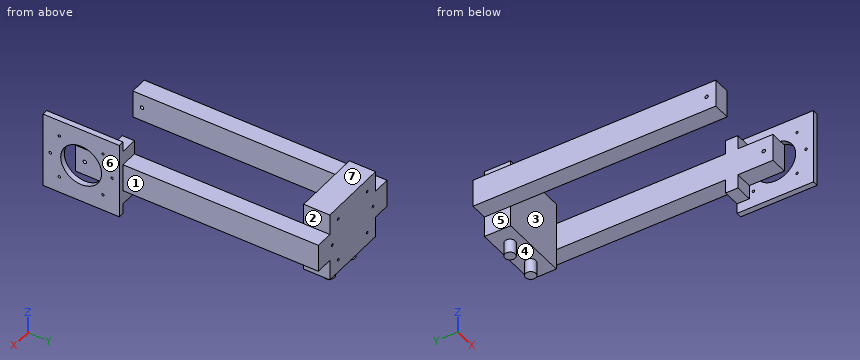
```python
from build123d import *

# Parameters (mm, degrees)
SKETCH_1_W          = 150
SKETCH_1_H          = 40
EXTRUDE_1_DEPTH     = 350
CUT_EXTRUDE_3_REACH = 362.174
SKETCH_7_W          = 50
SKETCH_7_H          = 312.232580329
CUT_EXTRUDE_4_REACH = 383.314
SKETCH_8_R          = 2.5
EXTRUDE_START       = -20
SKETCH_12_W         = 100
SKETCH_12_H         = 37.767419671
EXTRUDE_2_DEPTH     = 50
SKETCH_14_R         = 1.75
CUT_EXTRUDE_7_DEPTH = 25
SKETCH_16_R         = 7.5
EXTRUDE_3_DEPTH     = 20
SKETCH_18_W         = 110
SKETCH_18_H         = 110
EXTRUDE_4_DEPTH     = 8
SKETCH_19_R         = 1.75
CUT_EXTRUDE_8_DEPTH = 8
SKETCH_20_R         = 29.5
CUT_EXTRUDE_9_DEPTH = 8
SKETCH_21_W         = 20.347444736
SKETCH_21_H         = 17.71885043
EXTRUDE_5_DEPTH     = 25


with BuildPart() as part:
    # 草图1 → 凸台-拉伸1 (new body)
    with BuildSketch(Plane(origin=(0, 0, 0), x_dir=(1, 0, 0), z_dir=(0, 1, 0))):
        Rectangle(SKETCH_1_W, SKETCH_1_H)
    extrude(amount=EXTRUDE_1_DEPTH)

    # 草图7 → 切除-拉伸3 (cut, up to next)
    with BuildSketch(Plane(origin=(0, 0, -20), x_dir=(-1, 0, 0), z_dir=(0, 0, -1)), mode=Mode.PRIVATE) as cut_extrude_3_sk1:
        with Locations((-25, 156.116290165)):
            Rectangle(SKETCH_7_W, SKETCH_7_H)
    cut_extrude_3_tool1 = extrude(cut_extrude_3_sk1.sketch, amount=-CUT_EXTRUDE_3_REACH, mode=Mode.PRIVATE) & part.part
    cut_extrude_3 = cut_extrude_3_tool1.solids().sort_by_distance((25, 156.11629, -20))[0]
    add(cut_extrude_3, mode=Mode.SUBTRACT)

    # 镜向2: 切除-拉伸3 across plane
    add(cut_extrude_3.mirror(Plane(origin=(0, 0, 0), x_dir=(0, 0, 1), z_dir=(1, 0, 0))), mode=Mode.SUBTRACT)

    # 草图8 → 切除-拉伸4 (cut, up to next)
    with BuildSketch(Plane.ZY.offset(75), mode=Mode.PRIVATE) as cut_extrude_4_sk1:
        with Locations((0, 13.236112216)):
            Circle(SKETCH_8_R)
    cut_extrude_4_tool1 = extrude(cut_extrude_4_sk1.sketch, amount=-CUT_EXTRUDE_4_REACH, mode=Mode.PRIVATE) & part.part
    cut_extrude_4 = cut_extrude_4_tool1.solids().sort_by_distance((-75, 13.236112, 0))[0]
    add(cut_extrude_4, mode=Mode.SUBTRACT)

    # 镜向3: 切除-拉伸4 across plane
    add(cut_extrude_4.mirror(Plane(origin=(0, 0, 0), x_dir=(0, 0, 1), z_dir=(1, 0, 0))), mode=Mode.SUBTRACT)

    # 草图12 → 凸台-拉伸2 (add, symmetric)
    with BuildSketch(Plane.XY.offset(20).offset(EXTRUDE_START)):
        with Locations((0, 331.116290165)):
            Rectangle(SKETCH_12_W, SKETCH_12_H)
    extrude(amount=EXTRUDE_2_DEPTH, both=True)

    # 草图14 → 切除-拉伸7 (cut)
    with BuildSketch(Plane(origin=(0, 350, 0), x_dir=(1, 0, 0), z_dir=(0, 1, 0))):
        with Locations(Location((-31.466251763, -31.466251763, 0), (0, 0, 270))):
            Circle(SKETCH_14_R)
        with Locations(Location((-44.5, 0, 0), (0, 0, 270))):
            Circle(SKETCH_14_R)
        with Locations(Location((-31.466251763, 31.466251763, 0), (0, 0, 270))):
            Circle(SKETCH_14_R)
        with Locations(Location((31.466251763, 31.466251763, 0), (0, 0, 270))):
            Circle(SKETCH_14_R)
        with Locations(Location((44.5, 0, 0), (0, 0, 270))):
            Circle(SKETCH_14_R)
        with Locations(Location((31.466251763, -31.466251763, 0), (0, 0, 270))):
            Circle(SKETCH_14_R)
    extrude(amount=-CUT_EXTRUDE_7_DEPTH, mode=Mode.SUBTRACT)

    # 草图16 → 凸台-拉伸3 (add)
    with BuildSketch(Plane(origin=(0, 0, -50), x_dir=(-1, 0, 0), z_dir=(0, 0, -1))):
        with Locations(Location((-22.5, 331.116290164, 0), (0, 0, 180))):
            Circle(SKETCH_16_R)
        with Locations(Location((22.5, 331.116290164, 0), (0, 0, 180))):
            Circle(SKETCH_16_R)
    extrude(amount=EXTRUDE_3_DEPTH)

    # 草图18 → 凸台-拉伸4 (add)
    with BuildSketch(Plane(origin=(75, 0, 0), x_dir=(0, 0, -1), z_dir=(1, 0, 0))):
        with Locations((0, 13.236112216)):
            Rectangle(SKETCH_18_W, SKETCH_18_H)
    extrude(amount=EXTRUDE_4_DEPTH)

    # 草图19 → 切除-拉伸8 (cut)
    with BuildSketch(Plane(origin=(83, 0, 0), x_dir=(0, 0, -1), z_dir=(1, 0, 0))):
        with Locations((0, -31.263887784)):
            Circle(SKETCH_19_R)
        with Locations((-31.466251763, -18.230139547)):
            Circle(SKETCH_19_R)
        with Locations((-31.466251763, 44.702363979)):
            Circle(SKETCH_19_R)
        with Locations((0, 57.736112216)):
            Circle(SKETCH_19_R)
        with Locations((31.466251763, 44.702363979)):
            Circle(SKETCH_19_R)
        with Locations((31.466251763, -18.230139547)):
            Circle(SKETCH_19_R)
    extrude(amount=-CUT_EXTRUDE_8_DEPTH, mode=Mode.SUBTRACT)

    # 草图20 → 切除-拉伸9 (cut)
    with BuildSketch(Plane(origin=(83, 0, 0), x_dir=(0, 0, -1), z_dir=(1, 0, 0))):
        with Locations((0, 13.236112216)):
            Circle(SKETCH_20_R)
    extrude(amount=-CUT_EXTRUDE_9_DEPTH, mode=Mode.SUBTRACT)

    # 草图21 → 凸台-拉伸5 (add)
    with BuildSketch(Plane.ZY.offset(-75)):
        with Locations((-30.173722368, 59.376687001)):
            Rectangle(SKETCH_21_W, SKETCH_21_H)
    extrude_5 = extrude(amount=EXTRUDE_5_DEPTH)

    # 镜向4: 凸台-拉伸5 across plane
    add(extrude_5.mirror(Plane.XY))


solid = part.part
```
The model under review builds one solid part; all positions refer to its coordinate system, in mm. Face numbers are marked on the shaded views. A direction names the side the tool comes from. Round coordinates to 2 decimals unless told otherwise and drop trailing zeros. Order: outer loops, then holes, each group sorted by start corner. A loop starts at its lowest first (then second) coordinate and runs counter-clockwise, first axis right, second up. Notation, with made-up numbers: (5, -33.5) - (61, -33.5) arc R23 ccw to (61, -22.5) - close; hole circle Ø2 at (89.25, -6.5). An arc over 180 degrees is marked (long way). Answer in a Markdown table with one row per item.
(1) Take a section at A-A on y = 187. Write out the cut boundary in (x, z).
Result set:
| item | result |
|---|---|
| outline | (-75, -20) - (-50, -20) - (-50, 20) - (-75, 20) - close; (50, -20) - (75, -20) - (75, 20) - (50, 20) - close |
(2) Take a section at C-C on z = -15.5. Write out the cut boundary in (x, y), plus the area to 3 significant figures.
Result set:
| item | result |
|---|---|
| outline | (-75, 0) - (-50, 0) - (-50, 312.23) - (50, 312.23) - (50, 0) - (75, 0) - (75, 38.34) - (83, 38.34) - (83, 68.24) - (75, 68.24) - (75, 350) - (-75, 350) - close; (75, -41.76) - (83, -41.76) - (83, -11.86) - (75, -11.86) - close |
| area | 21,800 mm2 |
(3) For line 1 (Y direction, x = 81, z = 0); line 2 (X direction, y = 87.5, z = 5); line 3 (X direction, y = 53, z = 24), list the stretches that pass through material, from the lowest coordinate up. Write a range as from..to.
Result set:
| item | result |
|---|---|
| line 1 | y = -41.76..-33.01, -29.51..-16.26, 42.74..55.99, 59.49..68.24 |
| line 2 | x = -75..-50, 50..75 |
| line 3 | x = 50..83 |
(4) Take a section at D-D on x = 38.5. Write out the cut boundary in (y, z).
Result set:
| item | result |
|---|---|
| outline | (312.23, -50) - (350, -50) - (350, 50) - (312.23, 50) - close |
(5) Mouldability with a two-part tool opening along X and no side actions: class the marked faces 4, 5, 6 and 7 as released by +X, released by -X, zero draft, split by the parting line, or undercut.
Result set:
| item | result |
|---|---|
| face 4 | undercut |
| face 5 | released by -X |
| face 6 | released by +X |
| face 7 | zero draft |
(6) Clearance check with flat-ended pins moving along their axes: P1, Ø8, axis at y = 31.5, z = 34.5, coming from the -X side; P2, Ø3, axis at x = 31, z = 30.5, coming from the +Y side; P3, Ø3, axis at y = 13.24, z = 0, coming from the +X side; P4, Ø8, axis at x = 48, z = -39, coming from the -Y side. State where each tip first meets the part, or that it passes through.
Result set:
| item | result |
|---|---|
| P1 | stops at x = 75 |
| P2 | stops at y = 350 |
| P3 | passes through |
| P4 | stops at y = 50.52 |
(7) Machinability: for the marked faces 1, 2 and 3, which of the approach directions +Z, -Z, +X, -X, +Y, -Y give a long, thin tool a straight path to every point of the face, cutting with its end or side? Answer none if there is none.
Result set:
| item | result |
|---|---|
| face 1 | +Z, -Z, +X, +Y |
| face 2 | +Z, +X, +Y |
| face 3 | +Z, -Z, -Y |
(8) Take a section at B-B on x = -22.5. Write out the cut boundary in (y, z), plus the area to 3 significant figures.
Result set:
| item | result |
|---|---|
| outline | (312.23, -50) - (323.62, -50) - (323.62, -70) - (338.62, -70) - (338.62, -50) - (350, -50) - (350, 50) - (312.23, 50) - close |
| area | 4,080 mm2 |
